Verification items for the finished model (mm, model axes). Face numbers are marked on the shaded views. A direction names the side the tool comes from. Coordinates: 2 decimals unless noted, no trailing zeros. Order: outer loops, then holes, each group sorted by start corner. A loop starts at its lowest first (then second) coordinate and runs counter-clockwise, first axis right, second up.
Q1. Cross-section at C-C, the plane z = 2.75. Count the separate pieces of the cut face and the enclosed holes in it, and give its area (3 significant figures).
Q2. Draft check along Y on the marked faces 1, 2 and 3. Enter one of: pulls with the +Y half, pulls with the -Y half, needs draft (parallel to the pull), parting line crosses it, or undercut.
Q3. Cross-section at B-B, the plane x = -7.25. Record the boundary of the cut face in (y, z).
Q4. Set-up check for the marked faces 4 and 5: record each of +Z, -Z, +X, -X, +Y, -Y from which the full face is reachable in a straight line by a thin tool's end or side.
Q5. Thickness scan on line 1 (Y direction, x = 6, z = -7.5); line 2 (Y direction, x = -2.25, z = 2.75); line 3 (Y direction, x = 0.25, z = -9.5). Record the ranges inside material, lowest first.
Q6. Depth check by flat-ended pin: P1, Ø10, axis at x = -4.5, z = -8, coming from the -Y side; P2, Ø1.5, axis at x = 0.5, z = -9, coming from the -Y side; P3, Ø10, axis at x = -5.5, z = -9.5, coming from the -Y side. Enter the tip coordinate at first touch or a pass-through.
Q7. Cross-section at A-A, the plane y = 0. Record the boundary of the cut face in (x, z), and give its area (3 significant figures).
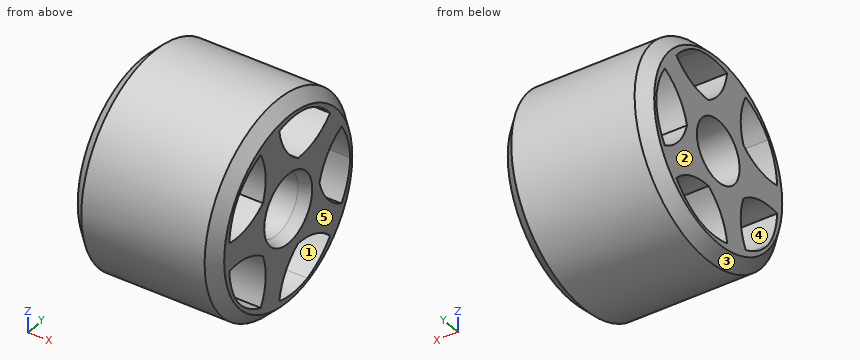
from build123d import *

# Parameters (mm, degrees)
SKETCH1_R           = 13.5
SKETCH1_R_2         = 4
BOSS_EXTRUDE1_DEPTH = 9.5
CUT_EXTRUDE1_DEPTH  = 22.324868112
CIRPATTERN1_COUNT   = 5
CHAMFER1_SIZE       = 1.5
CHAMFER2_SIZE       = 0.5
CHAMFER2_SIZE2      = 1.5


with BuildPart() as part:
    # Sketch1 → Boss-Extrude1 (new, symmetric)
    with BuildSketch(Plane(origin=(0, 0, 0), x_dir=(0, 0, -1), z_dir=(1, 0, 0))):
        Circle(SKETCH1_R)
        Circle(SKETCH1_R_2, mode=Mode.SUBTRACT)
    extrude(amount=BOSS_EXTRUDE1_DEPTH, both=True)

    # Sketch2 → Cut-Extrude1 (cut, symmetric)
    with BuildSketch(Plane(origin=(0, 0, 0), x_dir=(0, 0, -1), z_dir=(1, 0, 0))):
        with BuildLine():
            ThreePointArc((0, 5.849695328), (-2.956289657, 7.377375059), (-5.012219469, 9.99397715))
            ThreePointArc((-5.012219469, 9.99397715), (-2.621563936, 11.159720287), (0, 11.6087119))
            ThreePointArc((0, 11.6087119), (2.621563936, 11.159720287), (5.012219469, 9.99397715))
            ThreePointArc((5.012219469, 9.99397715), (2.956289657, 7.377375059), (0, 5.849695328))
        make_face()
    cut_extrude1 = extrude(amount=CUT_EXTRUDE1_DEPTH, both=True, mode=Mode.SUBTRACT)

    # CirPattern1: Cut-Extrude1 ×5 about axis
    cirpattern1_axis = Axis((0, 0, 0), (1, 0, 0))
    for i in range(1, CIRPATTERN1_COUNT):
        add(cut_extrude1.rotate(cirpattern1_axis, i * 360 / CIRPATTERN1_COUNT), mode=Mode.SUBTRACT)

    # Chamfer1
    chamfer1_edges = [part.edges().sort_by_distance(p)[0] for p in [
        (-9.5, 0, 13.5),
        (9.5, 0, 13.5),
    ]]
    chamfer(chamfer1_edges, length=CHAMFER1_SIZE)

    # Chamfer2
    chamfer2_edges = [part.edges().sort_by_distance(p)[0] for p in [
        (9.5, 0, 4),
    ]]
    chamfer2_side = [part.faces().sort_by_distance(p)[0] for p in [
        (9.5, 0, 11.660588745),
    ]]
    chamfer(chamfer2_edges, length=CHAMFER2_SIZE, length2=CHAMFER2_SIZE2, reference=chamfer2_side[0])


solid = part.part
Check values:
1. separate pieces: 4
1. enclosed holes: 0
1. area: 213 mm2
2. face 1: undercut
2. face 2: needs draft
2. face 3: parting line crosses it
3. outline: circle Ø27 at (0, 0); hole (-11.03, -1.82) arc R9.39 ccw to (-9.39, -6.82) arc R9.39 ccw to (-5.14, -9.93) arc R7.84 ccw to (-4.73, -3.44) arc R7.84 ccw to start; hole (-11.03, 1.82) arc R7.84 ccw to (-4.73, 3.44) arc R7.84 ccw to (-5.14, 9.93) arc R9.39 ccw to (-9.39, 6.82) arc R9.39 ccw to start; hole circle Ø8 at (0, 0); hole (-1.68, -11.05) arc R9.39 ccw to (3.59, -11.04) arc R9.39 ccw to (7.86, -7.96) arc R7.84 ccw to (1.81, -5.56) arc R7.84 ccw to start; hole (-1.68, 11.05) arc R7.84 ccw to (1.81, 5.56) arc R7.84 ccw to (7.86, 7.96) arc R9.39 ccw to (3.59, 11.04) arc R9.39 ccw to start; hole (5.85, 0) arc R7.84 ccw to (9.99, -5.01) arc R9.39 ccw to (11.61, 0) arc R9.39 ccw to (9.99, 5.01) arc R7.84 ccw to start
4. face 4: +X, -X
4. face 5: +Z, -Z, +X, +Y, -Y
5. line 1: y = -11.22 to -8.82, -4.32 to -0.24, 7.38 to 11.22
5. line 2: y = -13.22 to -10.95, -5.73 to -2.9, 2.9 to 7.21, 11.12 to 13.22
5. line 3: y = -9.59 to -6.14, -4.93 to -1.3, 6.34 to 9.59
6. P1: stops at y = -13.16
6. P2: stops at y = -10.69
6. P3: stops at y = -12.73
7. outline: (-9.5, -12) - (-8, -13.5) - (8, -13.5) - (9.5, -12) - (9.5, -11.38) - (-9.5, -11.38) - close; (-9.5, -7.19) - (9.5, -7.19) - (9.5, -4.5) - (8, -4) - (-9.5, -4) - close; (-9.5, 4) - (8, 4) - (9.5, 4.5) - (9.5, 7.19) - (-9.5, 7.19) - close; (-9.5, 11.38) - (9.5, 11.38) - (9.5, 12) - (8, 13.5) - (-8, 13.5) - (-9.5, 12) - close
7. area: 197 mm2
